Geometry check sheet. Reference: the model listing, model coordinates, mm. A direction names the side the tool comes from. Coordinates: 2 decimals unless noted, no trailing zeros. Order: outer loops, then holes, each group sorted by start corner. A loop starts at its lowest first (then second) coordinate and runs counter-clockwise, first axis right, second up. Notation, with made-up numbers: (-3.75, -36.5) - (1.25, -36.5) arc R31 ccw to (1.25, 1.5) - close; hole circle Ø8 at (47, 60). An arc over 180 degrees is marked (long way). Return JSON: item names as keys, results as strings. Group by question number.
Item 1: Gauge pin test, flat ends, axial feed: pin 1 (3 mm diameter, centred on x = -710.5, z = 245.5, fed in from -Y); pin 2 (4 mm diameter, centred on y = 29.5, z = 340.5, fed in from -X); pin 3 (8 mm diameter, centred on x = -773, z = 216.5, fed in from -Y). Record the tip position at first contact, or that the pin passes through.
Item 2: Tool access check on faces 1 (the flat face through (-486, -12, 160)), 2 (the flat face through (25, -32.474, 197)), 3 (the flat face through (-935, 28.043, 74)). Record the directions out of +Z, -Z, +X, -X, +Y, -Y that give a thin tool (end or side, any length) a straight path to the whole face; none if there is none.
Item 3: Scan lines: probe 1 along X at (y, z) = (-39, 66); probe 2 along X at (y, z) = (21.5, 123); probe 3 along Z at (x, y) = (-497.5, -17). Record each from-to range of solid material in increasing order.
Item 4: Section check D-D on x = -903.5. Enter the section's corners in (y, z).
Item 5: Section check B-B on y = -4. Enter the section's corners in (x, z).
Item 6: Section check A-A on z = 282.5. Enter the section's corners in (x, y), then the cut area to 3 significant figures.
Item 7: Section check C-C on z = 210.5. Enter the section's corners in (x, y), then the cut area to 3 significant figures.
from build123d import *

# Parameters (mm, degrees)
BOSS_EXTRUDE1_DEPTH = 400
BOSS_EXTRUDE2_DEPTH = 470


with BuildPart() as part:
    # Sketch1 → Boss-Extrude1 (new body)
    with BuildSketch(Plane.XY):
        Polygon((10.586659127, 38.043305377), (10.586659127, -32.473936002), (40.586659127, -32.473936002), (40.586659127, -42.473936002), (-9.413340873, -41.956694623), (-9.413340873, 28.043305377), (-39.413340873, 28.043305377), (-39.413340873, 38.043305377), align=None)
    boss_extrude1 = extrude(amount=BOSS_EXTRUDE1_DEPTH)

    # Sketch2 → Boss-Extrude2 (add)
    with BuildSketch(Plane.ZY.offset(9.413340873)):
        Polygon((150, 28.043305377), (250, 28.043305377), (250, -41.956694623), (240, -41.956694623), (240, 18.043305377), (160, 18.043305377), (160, -41.956694623), (150, -41.956694623), align=None)
    boss_extrude2 = extrude(amount=BOSS_EXTRUDE2_DEPTH)

    # Mirror2: Boss-Extrude2 across plane
    add(boss_extrude2.mirror(Plane.ZY.offset(479.413340873)))

    # Mirror3: Boss-Extrude1 across plane
    add(boss_extrude1.mirror(Plane.ZY.offset(479.413340873)))


solid = part.part
Computed:
{
 "1": {"pin 1": "stops at y = -41.96", "pin 2": "stops at x = -969.41", "pin 3": "stops at y = 18.04"},
 "2": {"face 1": "-Y", "face 2": "+Z, -Z, +X, +Y", "face 3": "-Z, -Y"},
 "3": {"probe 1": "x = -999.41 to -949.41, -9.41 to 40.59", "probe 2": "x = -969.41 to -949.41, -9.41 to 10.59", "probe 3": "z = 150 to 160, 240 to 250"},
 "4": {"outline": "(-41.96, 150) - (28.04, 150) - (28.04, 250) - (-41.96, 250) - (-41.96, 240) - (18.04, 240) - (18.04, 160) - (-41.96, 160) - close"},
 "5": {"outline": "(-969.41, 0) - (-949.41, 0) - (-949.41, 150) - (-9.41, 150) - (-9.41, 0) - (10.59, 0) - (10.59, 400) - (-9.41, 400) - (-9.41, 250) - (-949.41, 250) - (-949.41, 400) - (-969.41, 400) - close; hole (-949.41, 160) - (-9.41, 160) - (-9.41, 240) - (-949.41, 240) - close"},
 "6": {"outline": "(-999.41, -42.47) - (-949.41, -41.96) - (-949.41, 28.04) - (-919.41, 28.04) - (-919.41, 38.04) - (-969.41, 38.04) - (-969.41, -32.47) - (-999.41, -32.47) - close; (-39.41, 28.04) - (-9.41, 28.04) - (-9.41, -41.96) - (40.59, -42.47) - (40.59, -32.47) - (10.59, -32.47) - (10.59, 38.04) - (-39.41, 38.04) - close", "area": "4,390 mm²"},
 "7": {"outline": "(-999.41, -42.47) - (-949.41, -41.96) - (-949.41, 18.04) - (-9.41, 18.04) - (-9.41, -41.96) - (40.59, -42.47) - (40.59, -32.47) - (10.59, -32.47) - (10.59, 38.04) - (-39.41, 38.04) - (-39.41, 28.04) - (-919.41, 28.04) - (-919.41, 38.04) - (-969.41, 38.04) - (-969.41, -32.47) - (-999.41, -32.47) - close", "area": "13,800 mm²"}
}
